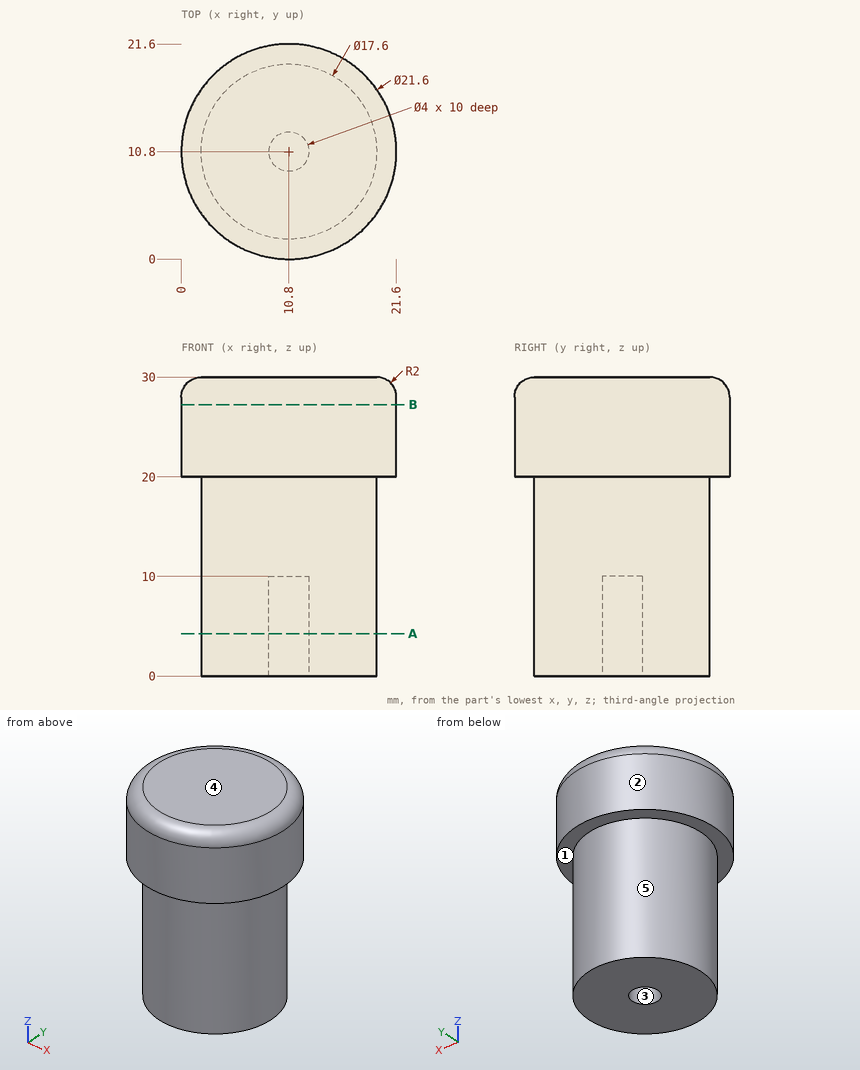
Print and shaded views of the part. All mm, measured from the part's lowest x, y and z. A direction names the side the tool comes from. Round coordinates to 2 decimals unless told otherwise and drop trailing zeros. Loops run counter-clockwise (first coordinate to the right, second up) from the corner with the lowest first, then second, coordinate; pieces in that order, holes last. Notation, with made-up numbers: M -30.5,-7.75 L 6.5,-7.75 A32 ccw 6.5,18.25 Z; hole C 71.25,40 d11. An arc over 180 degrees is marked long. One line per question, with ' | ' between items.
1) Band-saw the part on B-B (z = 27.25). Give the cut face in (x, y), then the cut area to 3 significant figures.
Solved:
outline: C 10.8,10.8 d21.6 | area: 366 mm²
2) 3-axis set-ups, long thin cutter, end or side, ignore diameter. For the marked faces 4 and 5: which of +Z, -Z, +X, -X, +Y, -Y reach the whole face in a straight line?
Solved:
face 4: +Z, +X, -X, +Y, -Y | face 5: -Z
3) Flat gauge pins, fed straight in: pin 1 (6 mm diameter, centred on x = 14, z = 15, fed in from -Y); pin 2 (1.5 mm diameter, centred on y = 4.5, z = 15.5, fed in from +X); pin 3 (4 mm diameter, centred on x = 15, z = 4.5, fed in from +Y). Where does each tip first touch, or does it go through?
Solved:
pin 1: stops at y = 2 | pin 2: stops at x = 17.63 | pin 3: stops at y = 19.32
4) Band-saw the part on A-A (z = 4.25). Give the cut face in (x, y), then the cut area to 3 significant figures.
Solved:
outline: C 10.8,10.8 d17.6; hole C 10.8,10.8 d4 | area: 231 mm²
5) Drill centre lines: line 1 along Y through (x, z) = (10.8, 6.5); line 2 along X through (y, z) = (12.5, 3.75); line 3 along Y through (x, z) = (12.25, 7.75). Where is each one in solid material? Low to high.
Solved:
line 1: y = 2 to 8.8, 12.8 to 19.6 | line 2: x = 2.17 to 9.75, 11.85 to 19.43 | line 3: y = 2.12 to 9.42, 12.18 to 19.48
6) Mould opens along X. For the marked faces 1, 2 and 3 say: +X half, -X half, draft (parallel to the pull), parting line (faces both ways), or undercut.
Solved:
face 1: draft | face 2: parting line | face 3: undercut
